from build123d import *

# Parameters (mm, degrees)
CROQUIS1_R              = 13
CROQUIS1_R_2            = 10
SALIENTE_EXTRUIR1_DEPTH = 50
CROQUIS2_W              = 2.444322312
CROQUIS2_H              = 0.823480184
SALIENTE_EXTRUIR2_DEPTH = 50


with BuildPart() as part:
    # Croquis1 → Saliente-Extruir1 (new body)
    with BuildSketch(Plane(origin=(0, 0, 0), x_dir=(1, 0, 0), z_dir=(0, 1, 0))):
        with Locations(Location((0, 0, 0), (0, 0, 270))):
            Circle(CROQUIS1_R)
        with Locations(Location((0, 0, 0), (0, 0, 270))):
            Circle(CROQUIS1_R_2, mode=Mode.SUBTRACT)
    extrude(amount=SALIENTE_EXTRUIR1_DEPTH)

    # Croquis2 → Saliente-Extruir2 (add)
    with BuildSketch(Plane(origin=(0, 50, 0), x_dir=(1, 0, 0), z_dir=(0, 1, 0))):
        with Locations((0, 13)):
            Rectangle(CROQUIS2_W, CROQUIS2_H)
    extrude(amount=-SALIENTE_EXTRUIR2_DEPTH)


solid = part.part
Geometry: final body of the model. Coordinates: model frame, mm. Coordinates: 2 decimals unless noted, no trailing zeros. Order: outer loops, then holes, each group sorted by start corner. A loop starts at its lowest first (then second) coordinate and runs counter-clockwise, first axis right, second up. Notation, with made-up numbers: (19, -11.5) - (65, -11.5) arc R29 ccw to (65, 8.5) - close; hole circle Ø5 at (-27, 40.25). An arc over 180 degrees is marked (long way). Use one line per item in the form item = value.
1) Section A-A (z = 0). Return loops of the section in (x, y).
Solutions:
outline = (-13, 0) - (-10, 0) - (-10, 50) - (-13, 50) - close; (10, 0) - (13, 0) - (13, 50) - (10, 50) - close
2) Pin query (flat end, axial travel): pin 1 (2 mm diameter, centred on x = -6, z = -10, fed in from -Y); pin 2 (2 mm diameter, centred on x = 7.5, y = 10.5, fed in from -Z); pin 3 (8 mm diameter, centred on y = 38.5, z = 9, fed in from -X); pin 4 (1.5 mm diameter, centred on x = -8.5, z = 1, fed in from -Y) (3 decimals). Return the tip coordinate at first contact, or that it passes through.
Solutions:
pin_1 = 0
pin_2 = -11.26
pin_3 = -12
pin_4 = through
3) Section D-D (z = -12). Return loops of the section in (x, y), then the cut area to 3 significant figures.
Solutions:
outline = (-5, 0) - (5, 0) - (5, 50) - (-5, 50) - close
area = 500 mm^2
4) Mould query, pull axis X, two halves, no side actions, for faces 1 (the face through (-9.76, 24.65, -2.17)), 2 (the face through (-10, 0, 4)). Classes: +X half, -X half, draft (parallel to the pull), parting line (faces both ways), or undercut.
Solutions:
face_1 = undercut
face_2 = draft
5) Section B-B (y = 16). Return loops of the section in (x, z), then the cut area to 3 significant figures.
Solutions:
outline = (-1.22, -13.41) - (1.22, -13.41) - (1.22, -12.94) arc R13 ccw (long way) to (-1.22, -12.94) - close; hole circle Ø20 at (0, 0)
area = 218 mm^2
6) Section C-C (x = -6.25). Return loops of the section in (y, z).
Solutions:
outline = (0, -11.4) - (50, -11.4) - (50, -7.81) - (0, -7.81) - close; (0, 7.81) - (50, 7.81) - (50, 11.4) - (0, 11.4) - close
7) Ray query, L1, parallel to X at y = 30, z = 0; L2, parallel to X at y = 37.5, z = 8.5; L3, parallel to Z at x = 1.5, y = 47. Return the intervals inside material, ascending.
Solutions:
L1 = -13 to -10, 10 to 13
L2 = -9.84 to -5.27, 5.27 to 9.84
L3 = -12.91 to -9.89, 9.89 to 12.91
